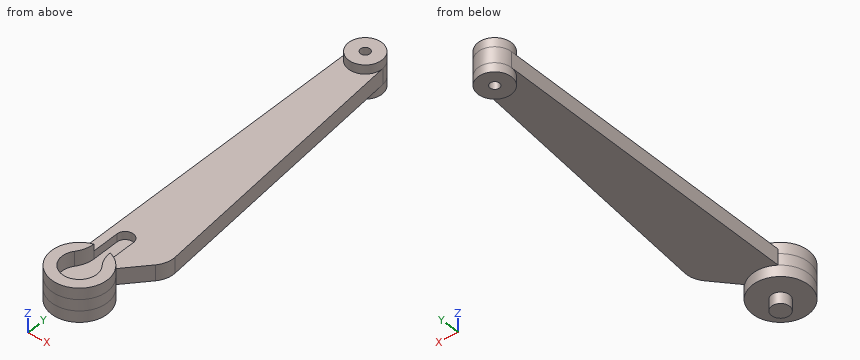
```python
from build123d import *
from build123d.topology import SkipClean

# Parameters (mm, degrees)
BOSS_EXTRUDE3_DEPTH     = 2.5
SKETCH3_R               = 12.4
BOSS_EXTRUDE5_DEPTH     = 5
BOSS_EXTRUDE8_START     = 5
SKETCH5_R               = 12.4
BOSS_EXTRUDE8_DEPTH     = 5
BOSS_EXTRUDE11_START    = 2
BOSS_EXTRUDE11_DEPTH    = 2
CUT_EXTRUDE3_DEPTH      = 4.5
CUT_EXTRUDE3_DEPTH_BACK = 2.5
BOSS_EXTRUDE12_START    = -7
BOSS_EXTRUDE12_DEPTH    = 7
FILLET1_R               = 10
SKETCH11_R              = 7.4
BOSS_EXTRUDE13_DEPTH    = 7.5
CUT_EXTRUDE6_DEPTH      = 6.55
SKETCH13_R              = 2.1
CUT_EXTRUDE7_DEPTH      = 160.423505726
SKETCH14_R              = 4
BOSS_EXTRUDE15_DEPTH    = 5


with BuildPart() as part:
    # Sketch1 → Boss-Extrude3 (new, symmetric)
    with BuildSketch(Plane.XY):
        with BuildLine():
            Line((7.4, 140.050125629), (7.4, 9.949874371))
            ThreePointArc((7.4, 9.949874371), (0, -12.4), (-7.4, 9.949874371))
            Line((-7.4, 9.949874371), (-7.4, 140.050125629))
            ThreePointArc((-7.4, 140.050125629), (0, 162.4), (7.4, 140.050125629))
        make_face()
    extrude(amount=BOSS_EXTRUDE3_DEPTH, both=True)

    # Sketch3 → Boss-Extrude5 (add)
    with BuildSketch(Plane(origin=(0, 0, -2.5), x_dir=(-1, 0, 0), z_dir=(0, 0, -1))):
        Circle(SKETCH3_R)
    extrude(amount=BOSS_EXTRUDE5_DEPTH)

    # Sketch5 → Boss-Extrude8 (add)
    with SkipClean():  # the faces are left unmerged after this step: merging them gives an invalid solid
        with BuildSketch(Plane.XY.offset(2.5).offset(BOSS_EXTRUDE8_START)):
            with Locations(Location((0, 0, 0), (0, 0, 180))):
                Circle(SKETCH5_R)
        extrude(amount=-BOSS_EXTRUDE8_DEPTH)

    # Sketch6 → Boss-Extrude11 (add)
    with SkipClean():  # the faces are left unmerged after this step: merging them gives an invalid solid
        with BuildSketch(Plane.XY.offset(2.5).offset(BOSS_EXTRUDE11_START)):
            with BuildLine():
                Line((7.4, 9.949874371), (7.4, 140.050125629))
                ThreePointArc((7.4, 140.050125629), (0, 137.6), (-7.4, 140.050125629))
                Line((-7.4, 140.050125629), (-7.4, 9.949874371))
                ThreePointArc((-7.4, 9.949874371), (0, 12.4), (7.4, 9.949874371))
            make_face()
            with BuildLine():
                ThreePointArc((-7.4, 140.050125629), (0, 137.6), (7.4, 140.050125629))
                ThreePointArc((7.4, 140.050125629), (11.079711188, 144.432235637), (12.4, 150))
                ThreePointArc((12.4, 150), (-5.567764363, 161.079711188), (-7.4, 140.050125629))
            make_face()
        extrude(amount=-BOSS_EXTRUDE11_DEPTH)

    # Sketch7 → Cut-Extrude3 (cut, two sides: drawn at the far end of the back side and taken through both)
    with SkipClean():  # the faces are left unmerged after this step: merging them gives an invalid solid
        with BuildSketch(Plane.XY.offset(-CUT_EXTRUDE3_DEPTH_BACK)):
            with BuildLine():
                ThreePointArc((-7.4, 140.050125629), (0, 162.4), (7.4, 140.050125629))
                Line((7.4, 140.050125629), (7.4, 134.868658063))
                Line((7.4, 134.868658063), (31.123214722, 134.868658063))
                Line((31.123214722, 134.868658063), (31.123214722, 164.335219314))
                Line((31.123214722, 164.335219314), (-28.315462738, 164.335219314))
                Line((-28.315462738, 164.335219314), (-28.315462738, 134.868658063))
                Line((-28.315462738, 134.868658063), (-7.4, 134.868658063))
                Line((-7.4, 134.868658063), (-7.4, 140.050125629))
            make_face()
            with BuildLine():
                Line((7.4, 150), (7.4, 140.050125629))
                ThreePointArc((7.4, 140.050125629), (0, 162.4), (-7.4, 140.050125629))
                Line((-7.4, 140.050125629), (-7.4, 150))
                ThreePointArc((-7.4, 150), (0, 157.4), (7.4, 150))
            make_face()
        extrude(amount=CUT_EXTRUDE3_DEPTH + CUT_EXTRUDE3_DEPTH_BACK, mode=Mode.SUBTRACT)

    # Sketch10 → Boss-Extrude12 (add)
    with SkipClean():  # the faces are left unmerged after this step: merging them gives an invalid solid
        with BuildSketch(Plane(origin=(0, 0, -2.5), x_dir=(-1, 0, 0), z_dir=(0, 0, -1)).offset(BOSS_EXTRUDE12_START)):
            with BuildLine():
                Line((-20, 22.981333294), (0, 0))
                Line((0, 0), (0, 12.4))
                ThreePointArc((0, 12.4), (-3.897534977, 11.771542851), (-7.4, 9.949874371))
                Line((-7.4, 9.949874371), (-7.4, 150))
                ThreePointArc((-7.4, 150), (-7.391010284, 150.364646378), (-7.364062978, 150.728406792))
                Line((-7.364062978, 150.728406792), (-20, 22.981333294))
            make_face()
        extrude(amount=BOSS_EXTRUDE12_DEPTH)

    # Fillet1
    fillet1_edges = [part.edges().sort_by_distance(p)[0] for p in [
        (20, 22.981333294, 1),
    ]]
    fillet(fillet1_edges, radius=FILLET1_R)

    # Sketch11 → Boss-Extrude13 (add, symmetric)
    with SkipClean():  # the faces are left unmerged after this step: merging them gives an invalid solid
        with BuildSketch(Plane.XY.offset(1)):
            with Locations((0, 150)):
                Circle(SKETCH11_R)
        extrude(amount=BOSS_EXTRUDE13_DEPTH, both=True)

    # Sketch12 → Cut-Extrude6 (cut)
    with SkipClean():  # the faces are left unmerged after this step: merging them gives an invalid solid
        with BuildSketch(Plane.XY.offset(7.5)):
            with BuildLine():
                Line((-3.65, 24), (-3.65, 12))
                ThreePointArc((-3.65, 12), (-4.285489279, 8.129790131), (-6.125220929, 4.666012063))
                ThreePointArc((-6.125220929, 4.666012063), (0, -7.7), (6.125220929, 4.666012063))
                ThreePointArc((6.125220929, 4.666012063), (4.285489279, 8.129790131), (3.65, 12))
                Line((3.65, 12), (3.65, 24))
                ThreePointArc((3.65, 24), (0, 27.65), (-3.65, 24))
            make_face()
        extrude(amount=-CUT_EXTRUDE6_DEPTH, mode=Mode.SUBTRACT)

    # Sketch13 → Cut-Extrude7 (cut, through all)
    with SkipClean():  # the faces are left unmerged after this step: merging them gives an invalid solid
        with BuildSketch(Plane.XY.offset(8.5)):
            with Locations((0, 150)):
                Circle(SKETCH13_R)
        extrude(amount=-CUT_EXTRUDE7_DEPTH, mode=Mode.SUBTRACT)

    # Sketch14 → Boss-Extrude15 (add)
    with SkipClean():  # the faces are left unmerged after this step: merging them gives an invalid solid
        with BuildSketch(Plane(origin=(0, 0, -7.5), x_dir=(-1, 0, 0), z_dir=(0, 0, -1))):
            Circle(SKETCH14_R)
        extrude(amount=BOSS_EXTRUDE15_DEPTH)


solid = part.part
```
The model under review builds one solid part; all positions refer to its coordinate system, in mm. Coordinates: 2 decimals unless noted, no trailing zeros. Order: outer loops, then holes, each group sorted by start corner. A loop starts at its lowest first (then second) coordinate and runs counter-clockwise, first axis right, second up. Notation, with made-up numbers: (5.25, 42.25) -> (29.25, 42.25) arc R19 cw to (29.25, 72.25) -> close; hole circle Ø4 at (-16, -14.5). An arc over 180 degrees is marked (long way). Answer in a Markdown table with one row per item. Add a question column.
Item 1: We need section B-B on y = 0. Write out the cut boundary in (x, z).
Item 2: We need section A-A on x = 0. Write out the cut boundary in (y, z).
Item 3: Clearance check with flat-ended pins moving along their axes: pin 1 (4.5 mm diameter, centred on x = 0, y = 150, fed in from -Z); pin 2 (6 mm diameter, centred on y = 102, z = -2, fed in from -X); pin 3 (6 mm diameter, centred on x = -6.5, y = 91.5, fed in from +Z); pin 4 (1 mm diameter, centred on x = -9, y = 39.5, fed in from -Z). State where each tip first meets the part, or that it passes through.
Item 4: To check wall thickness, follow probe 1 along Y at (x, z) = (0, 5); probe 2 along X at (y, z) = (150, 5.25); probe 3 along Y at (x, z) = (6.5, 5.75). State the ranges of each line that lie inside material, in increasing order.
Item 5: We need section D-D on y = 60. Write out the cut boundary in (x, z).
Item 6: We need section C-C on y = 33.5. Write out the cut boundary in (x, z).
Final values:
| question | item | result |
|---|---|---|
| 1 | outline | (-12.4, -7.5) -> (-4, -7.5) -> (-4, -12.5) -> (4, -12.5) -> (4, -7.5) -> (12.4, -7.5) -> (12.4, 7.5) -> (7.7, 7.5) -> (7.7, 0.95) -> (-7.7, 0.95) -> (-7.7, 7.5) -> (-12.4, 7.5) -> close |
| 2 | outline | (-12.4, -7.5) -> (-4, -7.5) -> (-4, -12.5) -> (4, -12.5) -> (4, -7.5) -> (12.4, -7.5) -> (12.4, -2.5) -> (142.6, -2.5) -> (142.6, -6.5) -> (147.9, -6.5) -> (147.9, 8.5) -> (142.6, 8.5) -> (142.6, 4.5) -> (27.65, 4.5) -> (27.65, 0.95) -> (-7.7, 0.95) -> (-7.7, 7.5) -> (-12.4, 7.5) -> close; (152.1, -6.5) -> (157.4, -6.5) -> (157.4, 8.5) -> (152.1, 8.5) -> close |
| 3 | pin 1 | stops at z = -6.5 |
| 3 | pin 2 | stops at x = -7.4 |
| 3 | pin 3 | stops at z = 4.5 |
| 3 | pin 4 | passes through |
| 4 | probe 1 | y = -12.4 to -7.7, 142.6 to 147.9, 152.1 to 157.4 |
| 4 | probe 2 | x = -7.4 to -2.1, 2.1 to 7.4 |
| 4 | probe 3 | y = -10.56 to -4.13, 4.13 to 10.56, 146.46 to 153.54 |
| 5 | outline | (-7.4, -2.5) -> (16.34, -2.5) -> (16.34, 4.5) -> (-7.4, 4.5) -> close |
| 6 | outline | (-7.4, -2.5) -> (18.96, -2.5) -> (18.96, 4.5) -> (-7.4, 4.5) -> close |
